Source: CAD feature listing. Evaluate the final solid. Frame: model axes, mm. A direction names the side the tool comes from. Round coordinates to 2 decimals unless told otherwise and drop trailing zeros. Write each loop counter-clockwise with the first axis right and the second up, starting at its lowest first coordinate (ties: lowest second). Pieces come first, ordered by that corner, then holes. Notation, with made-up numbers: M 82.25,52 L 103.25,52 A29 cw 103.25,79 Z; hole C -12,-3 d5. An arc over 180 degrees is marked long. Put each result on its own line as item: value. Start each with the question number.
```python
from build123d import *

# Parameters (mm, degrees)
BOSS_EXTRU_1_DEPTH      = 3
BOSS_EXTRU_2_DEPTH      = 15
ESQUISSE3_R             = 1.05
ENL_V_MAT_EXTRU_1_DEPTH = 6
ESQUISSE4_W             = 81
ESQUISSE4_H             = 15
BOSS_EXTRU_3_DEPTH      = 4
ESQUISSE5_R             = 1.5
ENL_V_MAT_EXTRU_2_DEPTH = 4


with BuildPart() as part:
    # Esquisse1 → Boss.-Extru.1 (new body)
    with BuildSketch(Plane.XY):
        Polygon((-12, 32), (-12, 28), (-6, 28), (-6, 32), (0, 32), (0, 0), (-18, 0), (-18, 32), align=None)
    extrude(amount=BOSS_EXTRU_1_DEPTH)

    # Esquisse2 → Boss.-Extru.2 (add)
    with BuildSketch(Plane.XY.offset(3)):
        Polygon((-18, 0), (0, 0), (0, 32), (-6, 32), (-6, 28), (-2.5, 28), (-2.5, 4), (-15.5, 4), (-15.5, 28), (-12, 28), (-12, 32), (-18, 32), align=None)
    extrude(amount=BOSS_EXTRU_2_DEPTH)

    # Esquisse3 → Enlèv. mat.-Extru.1 (cut)
    with BuildSketch(Plane.XY.offset(18)):
        with Locations((-9, 2.1)):
            Circle(ESQUISSE3_R)
    extrude(amount=-ENL_V_MAT_EXTRU_1_DEPTH, mode=Mode.SUBTRACT)

    # Esquisse4 → Boss.-Extru.3 (add)
    with BuildSketch(Plane.ZY.offset(18)):
        with Locations((15.5, 16)):
            Rectangle(ESQUISSE4_W, ESQUISSE4_H)
    extrude(amount=BOSS_EXTRU_3_DEPTH)

    # Esquisse5 → Enlèv. mat.-Extru.2 (cut)
    with BuildSketch(Plane.ZY.offset(22)):
        with Locations((-16, 16)):
            Circle(ESQUISSE5_R)
        with Locations((47, 16)):
            Circle(ESQUISSE5_R)
    extrude(amount=-ENL_V_MAT_EXTRU_2_DEPTH, mode=Mode.SUBTRACT)


solid = part.part
```
(1) Section query C-C (z = 2). Return loops of the section in (x, y), and give its area (3 significant figures).
(2) Access query for faces 4 (the flat face through (-14, 28, 10)), 5 (the flat face through (-18, 28, 9)), 6 (the flat face through (-18, 16, 37)), 7 (the flat face through (-18, 16, -13)). Directions: +Z, -Z, +X, -X, +Y, -Y. A direction counts if a zero-diameter tool reaches every point of the face in a straight line with its end or side. Return the directions, or none.
(3) Contact query for flat-ended pins moving along their axis: P1, Ø2.5, axis at x = -9, y = 2.1, coming from the -Z side; P2, Ø4.5, axis at x = -21, z = 23, coming from the +Y side; P3, Ø1.2, axis at y = 29.5, z = 12.5, coming from the -X side. Output: stop coordinate, or through.
(4) Ray query, line 1 along Y through (x, z) = (-3, 12); line 2 along X through (y, z) = (13.5, 9); line 3 along Z through (x, y) = (-13, 31.5). Return the intervals inside material, ascending.
(5) Section query B-B (z = -16). Return loops of the section in (x, y).
(6) Section query D-D (x = -9). Return loops of the section in (y, z).
(7) Section query A-A (y = 16). Return loops of the section in (x, z), and give its area (3 significant figures).
(8) Pull-direction query (Y, two-part tool) for faces 1 (the cylindrical face through (-20.03, 16.07, -17.5)), 2 (the flat face through (-20, 16, -25)), 3 (the flat face through (-3, 32, 9)); classes: +Y half, -Y half, draft (parallel to the pull), parting line (faces both ways), or undercut.
Entries:
1. outline: M -22,8.5 L -18,8.5 L -18,0 L 0,0 L 0,32 L -6,32 L -6,28 L -12,28 L -12,32 L -18,32 L -18,23.5 L -22,23.5 Z
1. area: 612 mm2
2. face 4: +Z
2. face 5: +Z, -Z, -X, +Y
2. face 6: +Z, +X, +Y, -Y
2. face 7: -Z, +X, +Y, -Y
3. P1: z = 0
3. P2: y = 23.5
3. P3: x = -18
4. line 1: 0 to 4, 28 to 32
4. line 2: -22 to -15.5, -2.5 to 0
4. line 3: 0 to 18
5. outline: M -22,8.5 L -18,8.5 L -18,14.5 L -22,14.5 Z; M -22,17.5 L -18,17.5 L -18,23.5 L -22,23.5 Z
6. outline: M 0,0 L 28,0 L 28,3 L 4,3 L 4,18 L 3.15,18 L 3.15,12 L 1.05,12 L 1.05,18 L 0,18 Z
7. outline: M -22,-25 L -18,-25 L -18,-17.5 L -22,-17.5 Z; M -22,-14.5 L -18,-14.5 L -18,0 L 0,0 L 0,18 L -2.5,18 L -2.5,3 L -15.5,3 L -15.5,18 L -18,18 L -18,45.5 L -22,45.5 Z; M -22,48.5 L -18,48.5 L -18,56 L -22,56 Z
7. area: 429 mm2
8. face 1: undercut
8. face 2: draft
8. face 3: +Y half
